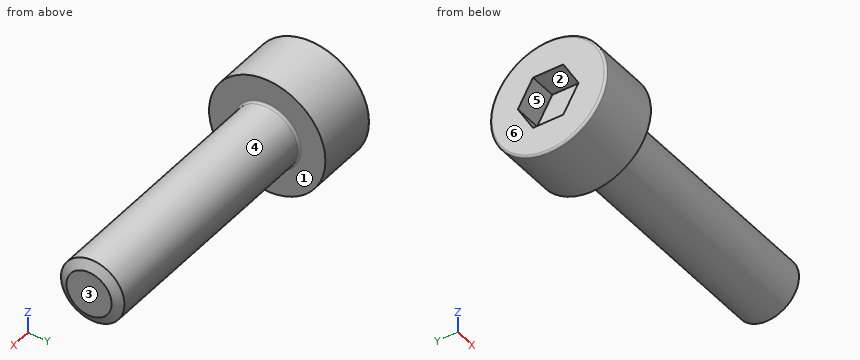
```python
from build123d import *

# Parameters (mm, degrees)
SKETCH_1_W          = 3
SKETCH_1_H          = 2.75
SKETCH_2_R          = 1.5
EXTRUDE_1_DEPTH     = 12
CUT_EXTRUDE_1_DEPTH = 1.3
CHAMFER_1_SIZE      = 0.433
CHAMFER_1_SIZE2     = 0.25
FILLET_1_R          = 0.1


with BuildPart() as part:
    # 草图1 → 旋转1 (revolve)
    with BuildSketch(Plane.XY):
        with Locations((1.5, 1.375)):
            Rectangle(SKETCH_1_W, SKETCH_1_H)
    revolve(axis=Axis((0, 0, 0), (1, 0, 0)))

    # 草图2 → 凸台-拉伸1 (add)
    with BuildSketch(Plane(origin=(3, 0, 0), x_dir=(0, 0, -1), z_dir=(1, 0, 0))):
        Circle(SKETCH_2_R)
    extrude(amount=EXTRUDE_1_DEPTH)

    # 草图3 → 切除-拉伸1 (cut)
    with BuildSketch(Plane.ZY):
        Polygon((0, 1.435), (-1.242746454, 0.7175), (-1.242746454, -0.7175), (0, -1.435), (1.242746454, -0.7175), (1.242746454, 0.7175), align=None)
    extrude(amount=-CUT_EXTRUDE_1_DEPTH, mode=Mode.SUBTRACT)

    # 倒角1
    chamfer_1_edges = [part.edges().sort_by_distance(p)[0] for p in [
        (15, 0, 1.5),
    ]]
    chamfer_1_side = [part.faces().sort_by_distance(p)[0] for p in [
        (15, 0, 0),
    ]]
    chamfer(chamfer_1_edges, length=CHAMFER_1_SIZE, length2=CHAMFER_1_SIZE2, reference=chamfer_1_side[0])

    # 圆角1
    fillet_1_edges = [part.edges().sort_by_distance(p)[0] for p in [
        (0, -2.75, 0),
        (3, 0, 1.5),
    ]]
    fillet(fillet_1_edges, radius=FILLET_1_R)


solid = part.part
```
Geometry check sheet. Reference: the model listing, model coordinates, mm. Face numbers are marked on the shaded views. A direction names the side the tool comes from. Round coordinates to 2 decimals unless told otherwise and drop trailing zeros. Order: outer loops, then holes, each group sorted by start corner. A loop starts at its lowest first (then second) coordinate and runs counter-clockwise, first axis right, second up. Notation, with made-up numbers: M 87.25,27 L 122.25,27 A5 cw 122.25,34 Z; hole C -33.5,17 d3. An arc over 180 degrees is marked long. Write item = value, one per line.
Q1. Depth check by flat-ended pin: pin 1 Ø2 at (y, z) = (0, 0) entering from -X; pin 2 Ø2 at (x, y) = (8, -1) entering from +Z; pin 3 Ø2 at (x, z) = (4.5, 0) entering from +Y; pin 4 Ø3 at (y, z) = (1, 0.5) entering from +X. Enter the tip coordinate at first touch or a pass-through.
Answer block:
pin_1 = 1.3
pin_2 = 1.5
pin_3 = 1.5
pin_4 = 15
Q2. Set-up check for the marked faces 1, 2 and 3: record each of +Z, -Z, +X, -X, +Y, -Y from which the full face is reachable in a straight line by a thin tool's end or side.
Answer block:
face_1 = +X
face_2 = -X
face_3 = +Z, -Z, +X, +Y, -Y
Q3. Scan lines: line 1 (X direction, y = -0.5, z = -1.8); line 2 (X direction, y = -0.2, z = 0.55); line 3 (Y direction, x = 8.5, z = -0.45). Record each from-to range of solid material in increasing order.
Answer block:
line_1 = 0 to 3
line_2 = 1.3 to 15
line_3 = -1.43 to 1.43
Q4. Section check A-A (y = 0). Enter the section's corners in (x, z), plus the area to 3 significant figures.
Answer block:
outline = M 0,-2.65 A0.1 ccw 0.1,-2.75 L 3,-2.75 L 3,-1.6 A0.1 cw 3.1,-1.5 L 14.75,-1.5 L 15,-1.07 L 15,1.07 L 14.75,1.5 L 3.1,1.5 A0.1 cw 3,1.6 L 3,2.75 L 0.1,2.75 A0.1 ccw 0,2.65 L 0,1.24 L 1.3,1.24 L 1.3,-1.24 L 0,-1.24 Z
area = 49.2 mm^2
Q5. Release check for a two-part mould opening along Y. For the marked faces 4, 5 and 6 record: released by +Y, released by -Y, zero draft, split by the parting line, or undercut.
Answer block:
face_4 = split by the parting line
face_5 = undercut
face_6 = zero draft
Q6. Section check B-B (x = 11). Enter the section's corners in (y, z), plus the area to 3 significant figures.
Answer block:
outline = C 0,0 d3
area = 7.07 mm^2
